Geometry: final body of the model. Coordinates: model frame, mm. A direction names the side the tool comes from. Round coordinates to 2 decimals unless told otherwise and drop trailing zeros. Loops run counter-clockwise (first coordinate to the right, second up) from the corner with the lowest first, then second, coordinate; pieces in that order, holes last. Notation, with made-up numbers: (-12.5, -35) - (2.5, -35) arc R32 ccw to (2.5, -1) - close; hole circle Ø11 at (-37.75, 9). An arc over 180 degrees is marked (long way). Use CSV: the item, a comma, the result in double quotes.
Autodesk Inventor part; units mm, degrees
ref_plane "rail25_to_dummy_XY" through (0, 0, 440) normal (0, 0, 1) x (1, 0, 0)
ref_plane "rail25_to_dummy_YZ" through (0, 0, 440) normal (1, 0, 0) x (0, 1, 0)
ref_plane "rail25_to_dummy_ZX" through (0, 0, 440) normal (0, 1, 0) x (0, 0, 1)
sketch "Sketch_1" plane through (0, 0, 0) normal (0, 0, 1) x (1, 0, 0)
  arc A0 (-12.5, 1) -> (-11.5, 0) centre (-11.5, 1) ccw
  line L0 (-11.5, 0) -> (11.5, 0)
  arc A1 (11.5, 0) -> (12.5, 1) centre (11.5, 1) ccw
  line L1 (12.5, 1) -> (12.5, 7.5)
  arc A2 (12.5, 7.5) -> (11.5, 8.5) centre (11.5, 7.5) ccw
  line L2 (11.5, 8.5) -> (9.5, 8.5)
  arc A3 (9.5, 8.5) -> (8.6036, 7.9432) centre (9.5, 7.5) ccw
  arc A4 (8.5, 3.4087) -> (8.6036, 7.9432) centre (7.5, 5.7) ccw
  line L3 (8.5, 3.4087) -> (8.5, 2.5)
  arc A5 (8, 2) -> (8.5, 2.5) centre (8, 2.5) ccw
  line L4 (8, 2) -> (-8, 2)
  arc A6 (-8.5, 2.5) -> (-8, 2) centre (-8, 2.5) ccw
  line L5 (-8.5, 2.5) -> (-8.5, 3.4087)
  arc A7 (-8.6036, 7.9432) -> (-8.5, 3.4087) centre (-7.5, 5.7) ccw
  arc A8 (-8.6036, 7.9432) -> (-9.5, 8.5) centre (-9.5, 7.5) ccw
  line L6 (-9.5, 8.5) -> (-11.5, 8.5)
  arc A9 (-11.5, 8.5) -> (-12.5, 7.5) centre (-11.5, 7.5) ccw
  line L7 (-12.5, 7.5) -> (-12.5, 1)
extrude "Extrusion1" add sketch "Sketch_1" along normal blind 310
sketch "Sketch_2" plane through (0, 0, 40) normal (0, 0, 1) x (1, 0, 0)
  line L0 (0, 0) -> (0, 2)
  line L1 (0, 2) -> (4.25, 2)
  line L2 (4.25, 2) -> (2.25, 0)
  line L3 (2.25, 0) -> (0, 0)
  line L4 (0, 0) -> (0, 2)
revolve "Revolution1" cut sketch "Sketch_2" angle 360 about axis through (0, 0, 40) along (0, -1, 0)
pattern_linear "Rectangular Pattern1" count 11 spacing 80 along (0, 0, 1) of "Revolution1"
sketch "Sketch_4" plane through (0, 2, 0) normal (0, 1, 0) x (1, 0, 0)
  circle A0 centre (0, -3) radius 5
extrude "Extrusion2" add sketch "Sketch_4" along normal blind 5
sketch "Sketch_5" plane through (0, 2, 0) normal (0, 1, 0) x (1, 0, 0)
  circle A0 centre (0, -877) radius 5
extrude "Extrusion3" [suppressed]
ref_plane "rail25_to_dummy_XY" through (0, 0, 440) normal (0, 0, 1) x (1, 0, 0)
ref_plane "rail25_to_dummy_YZ" through (0, 0, 440) normal (1, 0, 0) x (0, 1, 0)
ref_plane "rail25_to_dummy_ZX" through (0, 0, 440) normal (0, 1, 0) x (0, 0, 1)
ref_plane "to_slider_XY" through (0, 12, 440) normal (0, 0, 1) x (1, 0, 0)
ref_plane "to_slider_YZ" through (0, 12, 440) normal (1, 0, 0) x (0, 1, 0)
ref_plane "to_slider_ZX" through (0, 12, 440) normal (0, 1, 0) x (0, 0, 1)
properties part number "RSRR25-880"
Item 1: Section A-A on z = 280. Return the cut outline in (x, y).
Final values:
outline,"(-12.5, 1) arc R1 ccw to (-11.5, 0) - (-2.25, 0) - (-4.25, 2) - (-8, 2) arc R0.5 cw to (-8.5, 2.5) - (-8.5, 3.41) arc R2.5 cw to (-8.6, 7.94) arc R1 ccw to (-9.5, 8.5) - (-11.5, 8.5) arc R1 ccw to (-12.5, 7.5) - close; (2.25, 0) - (11.5, 0) arc R1 ccw to (12.5, 1) - (12.5, 7.5) arc R1 ccw to (11.5, 8.5) - (9.5, 8.5) arc R1 ccw to (8.6, 7.94) arc R2.5 cw to (8.5, 3.41) - (8.5, 2.5) arc R0.5 cw to (8, 2) - (4.25, 2) - close"
Item 2: Reachability of faces 1 (the flat face through (0, 7, 3)), 2 (the cylindrical face through (-0.651, 4.465, 7.957)), 3 (the flat face through (0, 2, 153)), 4 (the flat face through (0, 1, 0)) from +Z, -Z, +X, -X, +Y, -Y: full face, straight path, thin tool, end or side. Return the list, or none.
Final values:
face 1,"+Z, -Z, +Y"
face 2,"+Y"
face 3,"+Z, +Y"
face 4,"-Z, -Y"
Item 3: Pin query (flat end, axial travel): P1, Ø2, axis at x = 6.5, y = 7, coming from the +Z side; P2, Ø8, axis at x = -1.5, z = 189, coming from the +Y side; P3, Ø5, axis at x = 0.5, z = 2.5, coming from the +Y side; P4, Ø1, axis at x = -2.5, y = 4.5, coming from the +Z side. Return the tip coordinate at first contact, or that it passes through.
Final values:
P1,"passes through"
P2,"stops at y = 2"
P3,"stops at y = 7"
P4,"stops at z = 7.58"
Item 4: Section B-B on z = 3. Return the cut outline in (x, y), plus the area to 3 significant figures.
Final values:
outline,"(-12.5, 1) arc R1 ccw to (-11.5, 0) - (11.5, 0) arc R1 ccw to (12.5, 1) - (12.5, 7.5) arc R1 ccw to (11.5, 8.5) - (9.5, 8.5) arc R1 ccw to (8.6, 7.94) arc R2.5 cw to (8.5, 3.41) - (8.5, 2.5) arc R0.5 cw to (8, 2) - (5, 2) - (5, 7) - (-5, 7) - (-5, 2) - (-8, 2) arc R0.5 cw to (-8.5, 2.5) - (-8.5, 3.41) arc R2.5 cw to (-8.6, 7.94) arc R1 ccw to (-9.5, 8.5) - (-11.5, 8.5) arc R1 ccw to (-12.5, 7.5) - close"
area,"141 mm²"
Item 5: Section C-C on z = 103. Return the cut outline in (x, y).
Final values:
outline,"(-12.5, 1) arc R1 ccw to (-11.5, 0) - (11.5, 0) arc R1 ccw to (12.5, 1) - (12.5, 7.5) arc R1 ccw to (11.5, 8.5) - (9.5, 8.5) arc R1 ccw to (8.6, 7.94) arc R2.5 cw to (8.5, 3.41) - (8.5, 2.5) arc R0.5 cw to (8, 2) - (-8, 2) arc R0.5 cw to (-8.5, 2.5) - (-8.5, 3.41) arc R2.5 cw to (-8.6, 7.94) arc R1 ccw to (-9.5, 8.5) - (-11.5, 8.5) arc R1 ccw to (-12.5, 7.5) - close"
Item 6: Material intervals for line 1 (X direction, y = 7.25, z = 199); line 2 (X direction, y = 5.75, z = 149); line 3 (Z direction, x = 6, y = 1.5), sorted ascending.
Final values:
line 1,"x = -12.5 to -9.46, 9.46 to 12.5"
line 2,"x = -12.5 to -10, 10 to 12.5"
line 3,"z = 0 to 310"
